For this review, take the finished solid that the model builds, in its own axes (mm). Coordinates: 2 decimals unless noted, no trailing zeros. Loops run counter-clockwise (first coordinate to the right, second up) from the corner with the lowest first, then second, coordinate; pieces in that order, holes last.
1. To check wall thickness, follow probe 1 along Y at (x, z) = (3.5, -13.5); probe 2 along Z at (x, y) = (36, 24.5); probe 3 along Y at (x, z) = (33.5, -7). State the ranges of each line that lie inside material, in increasing order.
2. Take a section at A-A, the plane x = 29.5. State the section outline as (y, z) points.
3. Take a section at C-C, the plane z = -7.75. State the section outline as (x, y) points.
4. Take a section at B-B, the plane y = 17. State the section outline as (x, z) points, then the cut area to 3 significant figures.
5. Clearance check with a flat-ended pin moving along its axis: P1, Ø6, axis at x = 12, y = 28.5, coming from the +Z side. State where the tip first meets the part, or that it passes through.
```python
from build123d import *

# Parameters (mm, degrees)
F0_W     = 38.1
F0_H     = 33.02
F1_DEPTH = 25.4
F2_SIZE  = 5.08


with BuildPart() as f1:
    # F0 (on Top) → F1 (new body)
    with BuildSketch(Plane.XY):
        with Locations((19.05, 16.51)):
            Rectangle(F0_W, F0_H)
    extrude(amount=-F1_DEPTH)

    # F2
    f2_edges = [f1.edges().sort_by_distance(p)[0] for p in [
        (38.1, 0, -12.7),
        (38.1, 33.02, -12.7),
        (38.1, 16.51, -25.4),
        (19.05, 0, -25.4),
        (0, 0, -12.7),
        (19.05, 33.02, -25.4),
        (0, 33.02, -12.7),
        (0, 16.51, -25.4),
    ]]
    chamfer(f2_edges, length=F2_SIZE)


solid = f1.part
```
Results list:
1. probe 1: y = 1.58 to 31.44
1. probe 2: z = -22.42 to 0
1. probe 3: y = 0.48 to 32.54
2. outline: (0, -20.32) - (5.08, -25.4) - (27.94, -25.4) - (33.02, -20.32) - (33.02, 0) - (0, 0) - close
3. outline: (0, 5.08) - (5.08, 0) - (33.02, 0) - (38.1, 5.08) - (38.1, 27.94) - (33.02, 33.02) - (5.08, 33.02) - (0, 27.94) - close
4. outline: (0, -20.32) - (5.08, -25.4) - (33.02, -25.4) - (38.1, -20.32) - (38.1, 0) - (0, 0) - close
4. area: 942 mm2
5. P1: stops at z = 0
